Geometry: final body of the model. Coordinates: model frame, mm. Give positions to 0.01 mm unless a question says otherwise; leave off trailing zeros. Loops run counter-clockwise (first coordinate to the right, second up) from the corner with the lowest first, then second, coordinate; pieces in that order, holes last.
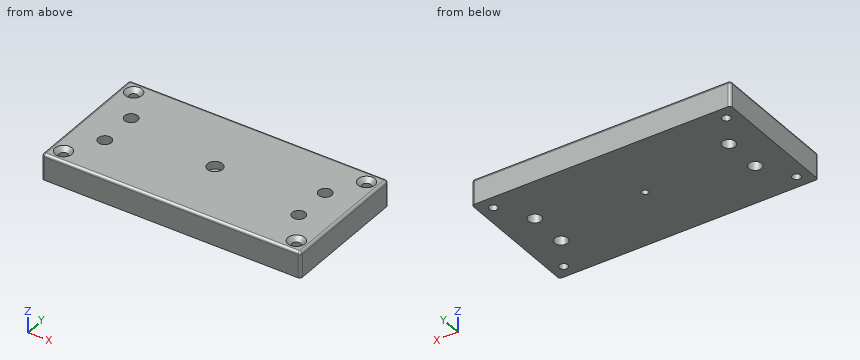
from build123d import *

# Parameters (mm, degrees)
F0_W           = 200
F0_H           = 100
F1_DEPTH       = 20
F2_R           = 5.05
F3_DEPTH       = 20.001
F5_D           = 6.5
F5_DEPTH       = 25
F5_CSINK_D     = 13
F5_CSINK_ANGLE = 90
F5_TIP         = 1.9527970118
F7_D           = 5
F7_DEPTH       = 20
F7_TIP         = 1.5021515476
F8_R           = 5.85
F8_R_2         = 2.5
F9_DEPTH       = 6
F10_R          = 2


with BuildPart() as f1:
    # F0 (on Top) → F1 (new body)
    with BuildSketch(Plane.XY):
        Rectangle(F0_W, F0_H)
    extrude(amount=F1_DEPTH)

    # F2 (on face) → F3 (cut, through all)
    with BuildSketch(Plane.XY.offset(20)):
        with Locations((-75, 15)):
            Circle(F2_R)
        with Locations((-75, -15)):
            Circle(F2_R)
        with Locations((75, -15)):
            Circle(F2_R)
        with Locations((75, 15)):
            Circle(F2_R)
    extrude(amount=-F3_DEPTH, mode=Mode.SUBTRACT)

    # F5
    with Locations(Plane.XY.offset(20)):
        with Locations((-90, 40), (90, 40), (90, -40), (-90, -40)):
            CounterSinkHole(F5_D / 2, F5_CSINK_D / 2, depth=F5_DEPTH, counter_sink_angle=F5_CSINK_ANGLE)
            with Locations((0, 0, -(F5_DEPTH + F5_TIP / 2))):  # 118° drill point
                Cone(0, F5_D / 2, F5_TIP, mode=Mode.SUBTRACT)

    # F7
    with Locations(Plane.XY.offset(20)):
        with Locations((0, 0)):
            Hole(F7_D / 2, depth=F7_DEPTH)
            with Locations((0, 0, -(F7_DEPTH + F7_TIP / 2))):  # 118° drill point
                Cone(0, F7_D / 2, F7_TIP, mode=Mode.SUBTRACT)

    # F8 (on face) → F9 (cut)
    with BuildSketch(Plane.XY.offset(20)):
        Circle(F8_R)
        Circle(F8_R_2, mode=Mode.SUBTRACT)
    extrude(amount=-F9_DEPTH, mode=Mode.SUBTRACT)

    # F10
    f10_edges = [f1.edges().sort_by_distance(p)[0] for p in [
        (-100, -50, 10),
        (100, -50, 10),
        (100, 50, 10),
        (-100, 50, 10),
        (0, 50, 20),
        (100, 0, 20),
        (0, -50, 20),
        (-100, 0, 20),
    ]]
    fillet(f10_edges, radius=F10_R)


solid = f1.part
Item 1: Section query C-C on x = -75. Return loops of the section in (y, z).
Values follow:
outline: (-50, 0) - (-20.05, 0) - (-20.05, 20) - (-48, 20) arc R2 ccw to (-50, 18) - close; (-9.95, 0) - (9.95, 0) - (9.95, 20) - (-9.95, 20) - close; (20.05, 0) - (50, 0) - (50, 18) arc R2 ccw to (48, 20) - (20.05, 20) - close
Item 2: Section query D-D on y = 0. Return loops of the section in (x, z), plus the area to 3 significant figures.
Values follow:
outline: (-100, 0) - (-2.5, 0) - (-2.5, 14) - (-5.85, 14) - (-5.85, 20) - (-98, 20) arc R2 ccw to (-100, 18) - close; (2.5, 0) - (100, 0) - (100, 18) arc R2 ccw to (98, 20) - (5.85, 20) - (5.85, 14) - (2.5, 14) - close
area: 3,860 mm2
Item 3: Section query A-A on y = -40. Return loops of the section in (x, z), plus the area to 3 significant figures.
Values follow:
outline: (-100, 0) - (-93.25, 0) - (-93.25, 16.75) - (-96.5, 20) - (-98, 20) arc R2 ccw to (-100, 18) - close; (-86.75, 0) - (86.75, 0) - (86.75, 16.75) - (83.5, 20) - (-83.5, 20) - (-86.75, 16.75) - close; (93.25, 0) - (100, 0) - (100, 18) arc R2 ccw to (98, 20) - (96.5, 20) - (93.25, 16.75) - close
area: 3,720 mm2
Item 4: Section query B-B on z = 6.75. Give the number of separate pieces and of enclosed holes in the cut face, plus the area to 3 significant figures.
Values follow:
separate pieces: 1
enclosed holes: 9
area: 19,500 mm2
Item 5: Ray query, probe 1 along Y at (x, z) = (90, 9.25); probe 2 along X at (y, z) = (-40, 11.75); probe 3 along Y at (x, z) = (75, 9). Return the intervals inside material, ascending.
Values follow:
probe 1: y = -50 to -43.25, -36.75 to 36.75, 43.25 to 50
probe 2: x = -100 to -93.25, -86.75 to 86.75, 93.25 to 100
probe 3: y = -50 to -20.05, -9.95 to 9.95, 20.05 to 50
Item 6: Pin query (flat end, axial travel): pin 1 (4 mm diameter, centred on x = -90, y = 40, fed in from +Z); pin 2 (10.5 mm diameter, centred on x = 0, y = 0, fed in from +Z). Return the tip coordinate at first contact, or that it passes through.
Values follow:
pin 1: passes through
pin 2: stops at z = 14
